Geometry check sheet. Reference: the model listing, model coordinates, mm. Face numbers are marked on the shaded views. Coordinates: 2 decimals unless noted, no trailing zeros. Write each loop counter-clockwise with the first axis right and the second up, starting at its lowest first coordinate (ties: lowest second). Pieces come first, ordered by that corner, then holes. Notation, with made-up numbers: M -28,-14.5 L 3,-14.5 A8 ccw 3,-6.5 Z; hole C 40,51 d4. An arc over 180 degrees is marked long. Put each result on its own line as item: value. Start each with the question number.
1) Mould release check, pull along Z, two halves, no side actions. Record for the marked faces 1, 2 and 3: released by +Z, released by -Z, zero draft, split by the parting line, or undercut.
2) Cross-section at A-A on y = 123.5. Record the cut outline in (x, z).
3) Gauge pin test, flat ends, axial feed: pin 1 (1 mm diameter, centred on y = 98, z = 28, fed in from +X); pin 2 (2 mm diameter, centred on x = -104.5, y = 134.5, fed in from +Z); pin 3 (3 mm diameter, centred on y = 101, z = 13.5, fed in from +X). Record the tip position at first contact, or that the pin passes through.
4) Cross-section at B-B on x = -113.5. Record the cut outline in (y, z), plus the area to 3 significant figures.
5) Cross-section at C-C on z = 28.5. Record the cut outline in (x, y).
6) Scan lines: line 1 along Z through (x, y) = (-127, 136.5); line 2 along X through (y, z) = (62, 15.5); line 3 along X through (y, z) = (119, 32.5). Record each from-to range of solid material in increasing order.
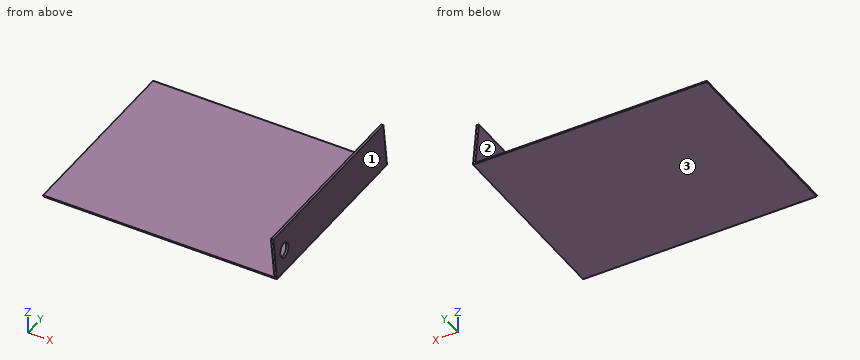
Autodesk Inventor part; units mm, degrees
ref_plane "YZ Plane" through (0, 0, 0) normal (1, 0, 0) x (0, 1, 0)
ref_plane "XZ Plane" through (0, 0, 0) normal (0, 1, 0) x (-1, 0, 0)
ref_plane "XY Plane" through (0, 0, 0) normal (0, 0, 1) x (1, 0, 0)
sketch "Sketch1" plane through (0, 0, 0) normal (0, 1, 0) x (-1, 0, 0)
  line L0 (0, 0) -> (5, 0)
  line L1 (5, 161) -> (0, 161)
  line L2 (0, 0) -> (197.574, 0)
  line L3 (197.574, 0) -> (197.574, 1)
  line L4 (197.574, 1) -> (0, 1)
  line L5 (0, 1) -> (0, 0)
  line L6 (0, 1) -> (3.0069, 35.3687)
  line L7 (0, 1) -> (34.5, 1) construction
  line L8 (3.0069, 35.3687) -> (1.0145, 35.543)
  line L9 (1.0145, 35.543) -> (-2.0951, 0)
  line L10 (-2.0951, 0) -> (0, 0)
  line L11 (197.574, 1) -> (197.3061, 0)
  line L12 (197.574, 1) -> (198.6093, 1) construction
  line L13 (3.0069, 35.3687) -> (0.9992, 35.3687)
  dimension "d1" = 5
  dimension "d2" = 197.574
  dimension "d3" = 1
  dimension "d4" = 34.5
  dimension "d5" = 85
  dimension "d6" = 2
  dimension "d11" = 105
extrude "Extrusion1" add sketch "Sketch1" along normal blind 161 contours L5 L4 L11 L2 L0 | L10 L9 L13 L6 L5 | L13 L9 L8
sketch "Sketch3" plane through (-3.0069, 0, 35.3687) normal (-0.9962, 0, -0.0872) x (-0.0872, 0, 0.9962)
  circle A0 centre (-17.9972, 13.5211) radius 6
  line L0 (-19.9848, 8.9507) -> (-15.1606, 8.9507)
  line L1 (-15.1606, 8.9507) -> (-15.1606, -1.5715)
  line L2 (-15.1606, -1.5715) -> (-19.9848, -1.5715)
  line L3 (-19.9848, -1.5715) -> (-19.9848, 8.9507)
  point P0 (-35.4962, 0)
  point P1 (-15.1606, 8.234)
  point P2 (-19.9848, 7.8599)
  dimension "d12" = 12
extrude "Extrusion3" cut sketch "Sketch3" against normal blind 58.2625 contours A0 L1 L0 L3 | L3 L0 L1 A0
properties part number "bottomCover"
Answer key:
1. face 1: released by +Z
1. face 2: undercut
1. face 3: released by -Z
2. outline: M -197.57,1 L -197.31,0 L 2.1,0 L -1.01,35.54 L -3.01,35.37 L 0,1 Z
3. pin 1: stops at x = -0.31
3. pin 2: stops at z = 1
3. pin 3: stops at x = 1.05
4. outline: M 0,0 L 161,0 L 161,1 L 0,1 Z
4. area: 161 mm²
5. outline: M -2.41,0 L -0.4,0 L -0.4,161 L -2.41,161 Z
6. line 1: z = 0 to 1
6. line 2: x = -1.27 to 0.74
6. line 3: x = -2.76 to -0.75
